Input: part model. Units: mm. Frame: model coordinates. Coordinates: 2 decimals unless noted, no trailing zeros. Loops run counter-clockwise (first coordinate to the right, second up) from the corner with the lowest first, then second, coordinate; pieces in that order, holes last. Notation, with made-up numbers: (67.25, 36) -> (83.25, 36) arc R21 ccw to (83.25, 68) -> close; hole circle Ø9 at (13, -13). An arc over 180 degrees is marked (long way). Answer as a JSON object with one key per item and string values.
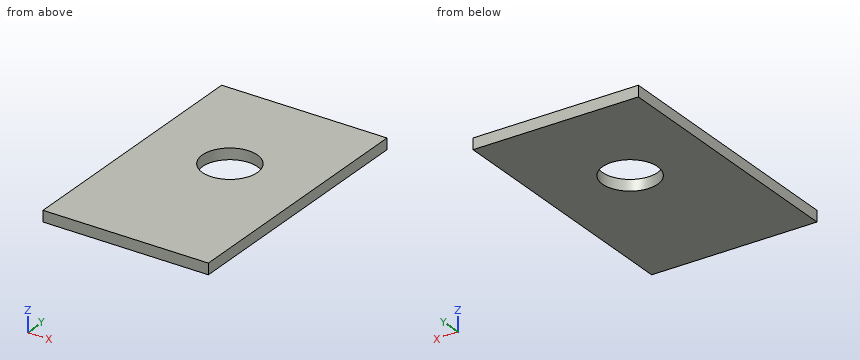
Autodesk Inventor part; units mm, degrees
ref_plane "XZ Plane" through (0, 0, 0) normal (0, 1, 0) x (-1, 0, 0)
ref_plane "XY Plane" through (0, 0, 0) normal (0, 0, 1) x (1, 0, 0)
sketch "Sketch1" plane through (0, 0, 0) normal (0, 0, 1) x (1, 0, 0)
  line L0 (-47.625, -76.2) -> (47.625, -76.2)
  line L1 (47.625, -76.2) -> (47.625, 76.2)
  line L2 (47.625, 76.2) -> (-47.625, 76.2)
  line L3 (-47.625, 76.2) -> (-47.625, -76.2)
  line L4 (-47.625, -76.2) -> (47.625, 76.2) construction
  line L5 (47.625, -76.2) -> (-47.625, 76.2) construction
  point P0 (0, 0)
  dimension "d0" = 95.25
  dimension "d1" = 152.4
extrude "Extrusion1" add sketch "Sketch1" against normal blind 6.35
sketch "Sketch2" plane through (0, 0, 0) normal (0, 0, 1) x (1, 0, 0)
  circle A0 centre (0, 12.7) radius 15.875
  line L0 (47.625, 76.2) -> (-47.625, 76.2)
  point P0 (0, 0)
  dimension "bearingDiameter" = 31.75
  dimension "d5" = 63.5
extrude "Extrusion2" cut sketch "Sketch2" against normal through all
properties part number "plateForHangingMechanism" material "Aluminum 6061"
1. Section query A-A (y = 12.7). Return loops of the section in (x, z) (3 decimals), plus the area to 3 significant figures.
Reply:
{"outline": "(-47.625, -6.35) -> (-15.875, -6.35) -> (-15.875, 0) -> (-47.625, 0) -> close; (15.875, -6.35) -> (47.625, -6.35) -> (47.625, 0) -> (15.875, 0) -> close", "area": "403 mm2"}
2. Line query: line 1 along Y through (x, z) = (0, -5) (3 decimals). Output: solid intervals per line, ascending.
Reply:
{"line 1": "y = -76.2 to -3.175, 28.575 to 76.2"}
3. Section query C-C (z = -1.75). Return loops of the section in (x, y) (3 decimals), plus the area to 3 significant figures.
Reply:
{"outline": "(-47.625, -76.2) -> (47.625, -76.2) -> (47.625, 76.2) -> (-47.625, 76.2) -> close; hole circle Ø31.75 at (0, 12.7)", "area": "13,700 mm2"}
4. Section query B-B (x = 0). Return loops of the section in (y, z) (3 decimals).
Reply:
{"outline": "(-76.2, -6.35) -> (-3.175, -6.35) -> (-3.175, 0) -> (-76.2, 0) -> close; (28.575, -6.35) -> (76.2, -6.35) -> (76.2, 0) -> (28.575, 0) -> close"}
